from build123d import *

# Parameters (mm, degrees)
SKETCH_R   = 1.6
SKETCH_R_2 = 1.1
PAD_DEPTH  = 4


with BuildPart() as part:
    # Sketch → Pad (new body)
    with BuildSketch(Plane.XY):
        with BuildLine():
            Line((7.5, 0), (7.5, 70))
            Line((7.5, 70), (20.227922, 82.727922))
            ThreePointArc((20.227922, 82.727922), (20.227922, 88.384776), (14.571068, 88.384776))
            Line((14.571068, 88.384776), (3.964466, 77.778175))
            Line((3.964466, 77.778175), (13.964466, 95.098683))
            ThreePointArc((13.964466, 95.098683), (12.500364, 100.562784), (7.036263, 99.098683))
            Line((0, 86.911518), (7.036263, 99.098683))
            Line((0, 86.911518), (0, 102))
            ThreePointArc((0, 102), (-4, 106), (-8, 102))
            Line((-8, 82), (-8, 102))
            Line((-14.211086, 95.319717), (-8, 82))
            ThreePointArc((-14.211086, 95.319717), (-19.52679, 97.254476), (-21.461549, 91.938771))
            Line((-12.163947, 72), (-21.461549, 91.938771))
            Line((-13.493151, 69.697751), (-12.163947, 72))
            Line((-13.493151, 69.697751), (-26.650635, 77.294229))
            ThreePointArc((-26.650635, 77.294229), (-32.797749, 75.647114), (-31.150635, 69.5))
            Line((-31.150635, 69.5), (-9.5, 57))
            Line((-13.312212, 13.348003), (-9.5, 57))
            ThreePointArc((-13.312212, 13.348003), (-13.110715, 11.701399), (-12.258507, 10.278146))
            Line((-12.258507, 10.278146), (-5.5, 3))
            Line((-5.5, 3), (-5.5, -5.09902))
            ThreePointArc((-5.5, -5.09902), (2.738613, -6.98212), (7.5, 0))
        make_face()
        Circle(SKETCH_R, mode=Mode.SUBTRACT)
        with Locations((-9.327379, 13)):
            Circle(SKETCH_R_2, mode=Mode.SUBTRACT)
    extrude(amount=PAD_DEPTH)


solid = part.part
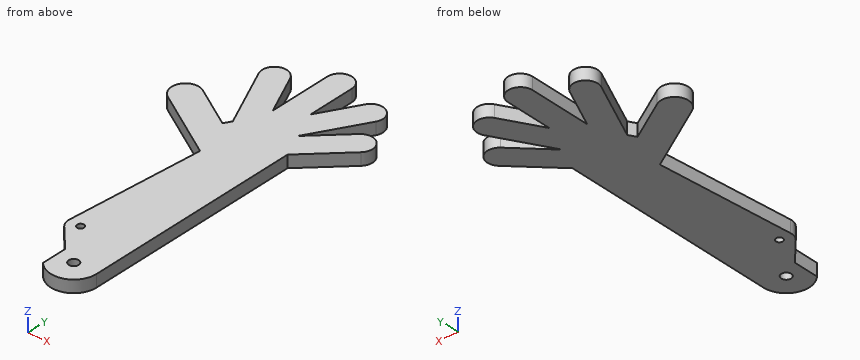
Geometry check sheet. Reference: the model listing, model coordinates, mm. Give positions to 0.01 mm unless a question says otherwise; leave off trailing zeros. Loops run counter-clockwise (first coordinate to the right, second up) from the corner with the lowest first, then second, coordinate; pieces in that order, holes last. Notation, with made-up numbers: M 74.5,60.5 L 126.5,60.5 A15 cw 126.5,66.5 Z; hole C 53,62.5 d9. An arc over 180 degrees is marked long. Write each question's results on one line, items separated by ' | '.
1) Section check D-D, the plane x = 17.5. Record the boundary of the cut face in (y, z), plus the area to 3 significant figures.
Answers follow:
outline: M 80,0 L 89.56,0 L 89.56,4 L 80,4 Z | area: 38.2 mm2
2) Section check C-C, the plane z = 1.3. Record the boundary of the cut face in (x, y).
Answers follow:
outline: M -31.15,69.5 L -9.5,57 L -13.31,13.35 A4 ccw -12.26,10.28 L -5.5,3 L -5.5,-5.1 A7.5 ccw 7.5,0 L 7.5,70 L 20.23,82.73 A4 ccw 14.57,88.38 L 3.96,77.78 L 13.96,95.1 A4 ccw 7.04,99.1 L 0,86.91 L 0,102 A4 ccw -8,102 L -8,82 L -14.21,95.32 A4 ccw -21.46,91.94 L -12.16,72 L -13.49,69.7 L -26.65,77.29 A4.5 ccw Z; hole C -9.33,13 d2.2; hole C 0,0 d3.2
3) Section check A-A, the plane x = -18.5. Record the boundary of the cut face in (y, z).
Answers follow:
outline: M 62.2,0 L 72.59,0 L 72.59,4 L 62.2,4 Z; M 85.59,0 L 97.57,0 L 97.57,4 L 85.59,4 Z
4) Section check B-B, the plane y = 80.5. Record the boundary of the cut face in (x, z).
Answers follow:
outline: M -16.13,0 L 5.54,0 L 5.54,4 L -16.13,4 Z; M 6.69,0 L 18,0 L 18,4 L 6.69,4 Z
5) Thickness scan on line 1 (X direction, y = 84, z = 3.5); line 2 (Y direction, x = -1, z = 2.6); line 3 (Y direction, x = 11.5, z = 3.25). Record the ranges inside material, lowest first.
Answers follow:
line 1: -17.76 to -8.93, -8 to 7.56, 10.19 to 21.08 | line 2: -7.43 to -1.25, 1.25 to 104.65 | line 3: 74 to 85.31, 90.83 to 100.97
6) Gauge pin test, flat ends, axial feed: pin 1 (1.2 mm diameter, centred on y = 93.5, z = 2.5, fed in from -X); pin 2 (1.2 mm diameter, centred on y = 51, z = 2, fed in from +X); pin 3 (1.2 mm diameter, centred on y = 93, z = 1, fed in from +X). Record the tip position at first contact, or that the pin passes through.
Answers follow:
pin 1: x = -21.84 | pin 2: x = 7.5 | pin 3: x = 13.1
